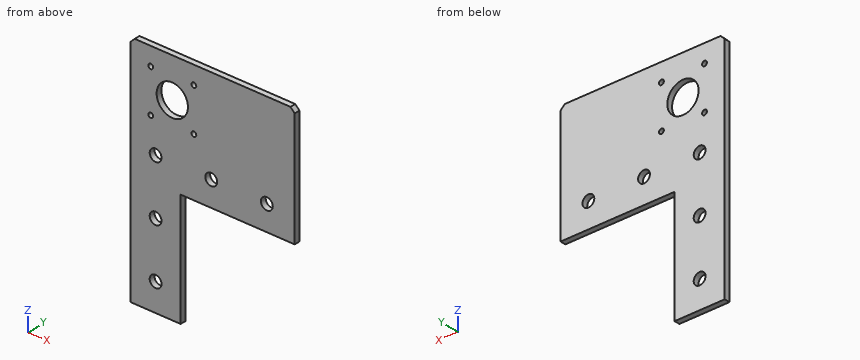
```python
from build123d import *

# Parameters (mm, degrees)
SKETCH1_R           = 4.25
BOSS_EXTRUDE1_DEPTH = 4
SKETCH1_3_R         = 1.75
SKETCH1_3_R_2       = 11.25
BOSS_EXTRUDE2_DEPTH = 4
CHAMFER1_SIZE       = 3


with BuildPart() as part:
    # Sketch1 → Boss-Extrude1 (new body)
    with BuildSketch(Plane(origin=(0, 0, 0), x_dir=(1, 0, 0), z_dir=(0, 1, 0))):
        Polygon((-30, 88), (-30, -30), (88, -30.072989915), (88, -30), (88, 6), (6, 6), (6, 88), align=None)
        with Locations(Location((-12, -12.011130611, 0), (0, 0, 270))):
            Circle(SKETCH1_R, mode=Mode.SUBTRACT)
        with Locations(Location((28, -12.011130611, 0), (0, 0, 270))):
            Circle(SKETCH1_R, mode=Mode.SUBTRACT)
        with Locations(Location((68, -12.011130611, 0), (0, 0, 270))):
            Circle(SKETCH1_R, mode=Mode.SUBTRACT)
        with Locations(Location((-12, 27.988869389, 0), (0, 0, 270))):
            Circle(SKETCH1_R, mode=Mode.SUBTRACT)
        with Locations(Location((-12, 67.988869389, 0), (0, 0, 270))):
            Circle(SKETCH1_R, mode=Mode.SUBTRACT)
    extrude(amount=BOSS_EXTRUDE1_DEPTH)

    # Sketch1_3 → Boss-Extrude2 (add)
    with BuildSketch(Plane(origin=(0, 0, 0), x_dir=(1, 0, 0), z_dir=(0, 1, 0))):
        Polygon((88, -30.072989915), (-30, -30), (-30, -80), (88, -80), align=None)
        with Locations(Location((-15.5, -67, 0), (0, 0, 270))):
            Circle(SKETCH1_3_R, mode=Mode.SUBTRACT)
        with Locations(Location((15.5, -67, 0), (0, 0, 270))):
            Circle(SKETCH1_3_R, mode=Mode.SUBTRACT)
        with Locations(Location((0, -51.5, 0), (0, 0, 270))):
            Circle(SKETCH1_3_R_2, mode=Mode.SUBTRACT)
        with Locations(Location((-15.5, -36, 0), (0, 0, 270))):
            Circle(SKETCH1_3_R, mode=Mode.SUBTRACT)
        with Locations(Location((15.5, -36, 0), (0, 0, 270))):
            Circle(SKETCH1_3_R, mode=Mode.SUBTRACT)
    extrude(amount=BOSS_EXTRUDE2_DEPTH)

    # Chamfer1
    chamfer1_edges = [part.edges().sort_by_distance(p)[0] for p in [
        (-30, 2, 80),
        (88, 2, 80),
    ]]
    chamfer(chamfer1_edges, length=CHAMFER1_SIZE)


solid = part.part
```
Check sheet for the modelled part. Datum: model origin and axes. Units: mm. Coordinates: 2 decimals unless noted, no trailing zeros. Order: outer loops, then holes, each group sorted by start corner. A loop starts at its lowest first (then second) coordinate and runs counter-clockwise, first axis right, second up. Notation, with made-up numbers: M 72.25,-30 L 108.25,-30 A20 cw 108.25,1 Z; hole C 75.5,63.25 d7. An arc over 180 degrees is marked long. One line per question, with ' | ' between items. Start each with the question number.
Item 1: Sectioned sample at B-B on y = 2.95. Count the separate pieces of the cut face and the enclosed holes in it, and give its area (3 significant figures).
Item 2: Sectioned sample at D-D on z = 36. Record the cut outline in (x, y).
Item 3: Gauge pin test, flat ends, axial feed: P1, Ø2, axis at y = 2.5, z = -44.5, coming from the +X side; P2, Ø3, axis at x = -15.5, z = 36, coming from the -Y side; P3, Ø2, axis at x = 68, y = 3.5, coming from the -Z side. Record the tip position at first contact, or that the pin passes through.
Item 4: Sectioned sample at C-C on x = 15.5. Record the cut outline in (y, z).
Item 5: Sectioned sample at A-A on x = 28. Record the cut outline in (y, z), and give its area (3 significant figures).
Item 6: Material ranges on line 1 (X direction, y = 2, z = 67); line 2 (X direction, y = 3.15, z = 51.5); line 3 (Z direction, x = -11.5, y = 2.65), recorded low to high.
Answer below:
1) separate pieces: 1 | enclosed holes: 10 | area: 12,400 mm^2
2) outline: M -30,0 L -17.25,0 L -17.25,4 L -30,4 Z; M -13.75,0 L 13.75,0 L 13.75,4 L -13.75,4 Z; M 17.25,0 L 88,0 L 88,4 L 17.25,4 Z
3) P1: stops at x = 6 | P2: passes through | P3: stops at z = -6
4) outline: M 0,-6 L 4,-6 L 4,34.25 L 0,34.25 Z; M 0,37.75 L 4,37.75 L 4,65.25 L 0,65.25 Z; M 0,68.75 L 4,68.75 L 4,80 L 0,80 Z
5) outline: M 0,-6 L 4,-6 L 4,7.76 L 0,7.76 Z; M 0,16.26 L 4,16.26 L 4,80 L 0,80 Z | area: 310 mm^2
6) line 1: x = -30 to -17.25, -13.75 to 13.75, 17.25 to 88 | line 2: x = -30 to -11.25, 11.25 to 88 | line 3: z = -88 to -72.21, -63.77 to -32.21, -23.77 to 7.79, 16.23 to 80
